Build history of the part. All positions in model axes, mm. Face numbers are marked on the shaded views. A direction names the side the tool comes from. Round coordinates to 2 decimals unless told otherwise and drop trailing zeros. Order: outer loops, then holes, each group sorted by start corner. A loop starts at its lowest first (then second) coordinate and runs counter-clockwise, first axis right, second up. Notation, with made-up numbers: (-19, -22) -> (27, -22) arc R32 ccw to (27, 12) -> close; hole circle Ø7 at (-4, 86). An arc over 180 degrees is marked (long way). Write item = value, one per line.
from build123d import *

# Parameters (mm, degrees)
SKETCH1_W           = 40
SKETCH1_H           = 40
BOSS_EXTRUDE1_DEPTH = 5
CUT_EXTRUDE2_DEPTH  = 39
SKETCH4_W           = 12
SKETCH4_H           = 6.7
CUT_EXTRUDE3_DEPTH  = 29.609264234
SKETCH5_W           = 6
SKETCH5_H           = 6
BOSS_EXTRUDE2_DEPTH = 1.7
FILLET1_R           = 1
SKETCH6_R           = 1
BOSS_EXTRUDE3_DEPTH = 0.5
FILLET2_R           = 1
SKETCH7_R           = 1.6
BOSS_EXTRUDE4_DEPTH = 5
FILLET3_R           = 3


with BuildPart() as part:
    # Sketch1 → Boss-Extrude1 (new body)
    with BuildSketch(Plane(origin=(0, 0, 0), x_dir=(1, 0, 0), z_dir=(0, 1, 0))):
        Rectangle(SKETCH1_W, SKETCH1_H)
    extrude(amount=BOSS_EXTRUDE1_DEPTH)

    # Sketch3 → Cut-Extrude2 (cut)
    with BuildSketch(Plane.XY.offset(20)):
        Polygon((-18.1, 5), (-18.1, 4.2), (-19.1, 4.2), (-19.1, 2.4), (-18.1, 2.4), (-18.1, 0.7), (18.1, 0.7), (18.1, 2.4), (19.1, 2.4), (19.1, 4.2), (18.1, 4.2), (18.1, 5), align=None)
    extrude(amount=-CUT_EXTRUDE2_DEPTH, mode=Mode.SUBTRACT)

    # Sketch4 → Cut-Extrude3 (cut, through all)
    with BuildSketch(Plane(origin=(0, 0.7, 0), x_dir=(1, 0, 0), z_dir=(0, 1, 0))):
        with Locations((8.6, -16.65)):
            Rectangle(SKETCH4_W, SKETCH4_H)
    extrude(amount=-CUT_EXTRUDE3_DEPTH, mode=Mode.SUBTRACT)

    # Sketch5 → Boss-Extrude2 (add)
    with BuildSketch(Plane(origin=(0, 0.7, 0), x_dir=(1, 0, 0), z_dir=(0, 1, 0))):
        with Locations((-15.1, 16)):
            Rectangle(SKETCH5_W, SKETCH5_H)
        with Locations((15.1, 16)):
            Rectangle(SKETCH5_W, SKETCH5_H)
    extrude(amount=BOSS_EXTRUDE2_DEPTH)

    # Fillet1
    fillet1_edges = [part.edges().sort_by_distance(p)[0] for p in [
        (2.6, 0.35, 20),
        (2.6, 0.35, 13.3),
        (14.6, 0.35, 13.3),
        (14.6, 0.35, 20),
        (-18.1, 1.55, -13),
        (-12.1, 1.55, -13),
        (-12.1, 1.55, -19),
        (18.1, 1.55, -13),
        (12.1, 1.55, -19),
        (12.1, 1.55, -13),
    ]]
    fillet(fillet1_edges, radius=FILLET1_R)

    # Sketch6 → Boss-Extrude3 (add)
    with BuildSketch(Plane(origin=(0, 2.4, 0), x_dir=(1, 0, 0), z_dir=(0, 1, 0))):
        with Locations((-17.1, 17)):
            Circle(SKETCH6_R)
        with Locations((17.1, 17)):
            Circle(SKETCH6_R)
    extrude(amount=BOSS_EXTRUDE3_DEPTH)

    # Fillet2
    # the kernel refuses this fillet: 1 mm, written as the material it takes off along each edge
    with BuildSketch(Plane(origin=(-17.1, 2.9, -17), x_dir=(1, 0, 0), z_dir=(0, 0, 1))) as fillet2_piece_1:
        with BuildLine():
            CenterArc((0.133974596, -1), FILLET2_R, 30, 60)
            Line((0.133974596, 0), (0.133974596, 0.02))
            Line((0.133974596, 0.02), (1, 0.02))
            Line((1, 0.02), (1.02, 0))
            ThreePointArc((1.02, 0), (1.02, -0.25), (1.017320508, -0.49))
            Line((1.017320508, -0.49), (1, -0.5))
        make_face()
    revolve(axis=Axis((-17.1, 2.9, -17), (0, 1, 0)), mode=Mode.SUBTRACT)
    with BuildSketch(Plane(origin=(17.1, 2.9, -17), x_dir=(1, 0, 0), z_dir=(0, 0, 1))) as fillet2_piece_2:
        with BuildLine():
            CenterArc((0.133974596, -1), FILLET2_R, 30, 60)
            Line((0.133974596, 0), (0.133974596, 0.02))
            Line((0.133974596, 0.02), (1, 0.02))
            Line((1, 0.02), (1.02, 0))
            ThreePointArc((1.02, 0), (1.02, -0.25), (1.017320508, -0.49))
            Line((1.017320508, -0.49), (1, -0.5))
        make_face()
    revolve(axis=Axis((17.1, 2.9, -17), (0, 1, 0)), mode=Mode.SUBTRACT)

    # Sketch7 → Boss-Extrude4 (add)
    # profile 1 of 2: a face of its own
    with BuildSketch(Plane.XZ):
        with BuildLine():
            Line((-20, 20), (-20, 11.521537766))
            Line((-20, 11.521537766), (-24.997516692, 14.400491632))
            ThreePointArc((-24.997516692, 14.400491632), (-26.398148125, 17.775072543), (-23.5, 20))
            Line((-23.5, 20), (-20, 20))
        make_face()
        with Locations(Location((-23.5, 17, 0), (0, 0, 270))):
            Circle(SKETCH7_R, mode=Mode.SUBTRACT)
    # profile 2 of 2: a face of its own
    with BuildSketch(Plane.XZ):
        with BuildLine():
            Line((20, -20), (20, -11.521537766))
            Line((20, -11.521537766), (24.997516692, -14.400491632))
            ThreePointArc((24.997516692, -14.400491632), (26.398148125, -17.775072543), (23.5, -20))
            Line((23.5, -20), (20, -20))
        make_face()
        with Locations(Location((23.5, -17, 0), (0, 0, 270))):
            Circle(SKETCH7_R, mode=Mode.SUBTRACT)
    extrude(amount=-BOSS_EXTRUDE4_DEPTH)

    # Fillet3
    fillet3_edges = [part.edges().sort_by_distance(p)[0] for p in [
        (-20, 2.5, 11.521537766),
        (20, 2.5, -11.521537766),
    ]]
    fillet(fillet3_edges, radius=FILLET3_R)


solid = part.part
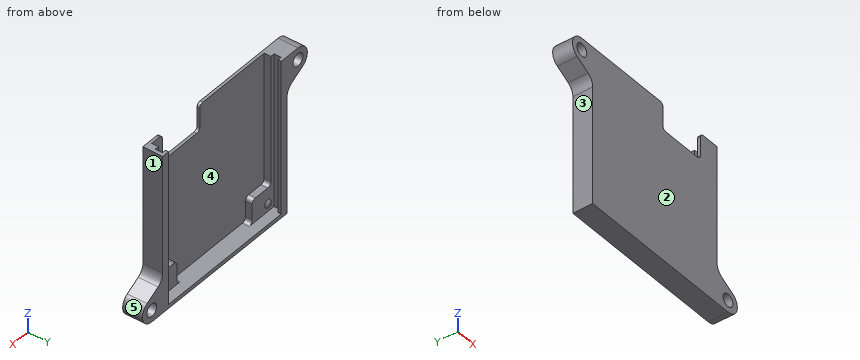
Q1. Which spindle directions (+Z, -Z, +X, -X, +Y, -Y) get a long thin tool onto all of the face, cutting with end or side? Do the marked faces 1, 2, 3, 4 and 5. Say none if no direction does.
Check values:
face_1 = +Z, +X, +Y, -Y
face_2 = +Z, -Z, +X, -X, -Y
face_3 = -Z, -X, +Y, -Y
face_4 = +Z, +Y
face_5 = +X, +Y, -Y
Q2. Cut at D-D, the plane z = -11. List the corners of the cut face in (x, y), and give its area (3 significant figures).
Check values:
outline = (-20, 0) -> (20.26, 0) -> (20.26, 5) -> (18.1, 5) -> (18.1, 4.2) -> (19.1, 4.2) -> (19.1, 2.4) -> (18.1, 2.4) -> (18.1, 0.7) -> (-18.1, 0.7) -> (-18.1, 2.4) -> (-19.1, 2.4) -> (-19.1, 4.2) -> (-18.1, 4.2) -> (-18.1, 5) -> (-20, 5) -> close
area = 42.0 mm²
Q3. Cut at B-B, the plane z = 5.5. List the corners of the cut face in (x, y), and give its area (3 significant figures).
Check values:
outline = (-20, 0) -> (20, 0) -> (20, 5) -> (18.1, 5) -> (18.1, 4.2) -> (19.1, 4.2) -> (19.1, 2.4) -> (18.1, 2.4) -> (18.1, 0.7) -> (-18.1, 0.7) -> (-18.1, 2.4) -> (-19.1, 2.4) -> (-19.1, 4.2) -> (-18.1, 4.2) -> (-18.1, 5) -> (-20, 5) -> close
area = 40.7 mm²
Q4. Cut at A-A, the plane z = 17. List the corners of the cut face in (x, y).
Check values:
outline = (-26.5, 0) -> (-25.1, 0) -> (-25.1, 5) -> (-26.5, 5) -> close; (-21.9, 0) -> (2.6, 0) -> (2.6, 0.7) -> (-18.1, 0.7) -> (-18.1, 2.4) -> (-19.1, 2.4) -> (-19.1, 4.2) -> (-18.1, 4.2) -> (-18.1, 5) -> (-21.9, 5) -> close; (14.6, 0) -> (20, 0) -> (20, 5) -> (18.1, 5) -> (18.1, 4.2) -> (19.1, 4.2) -> (19.1, 2.4) -> (18.1, 2.4) -> (18.1, 0.7) -> (14.6, 0.7) -> close
Q5. Probe probe 1 along X at (y, z) = (4.05, 17); probe 2 along X at (y, z) = (1.65, -17); probe 3 along X at (y, z) = (2, -2). List the from-to ranges inside material, lowest first.
Check values:
probe_1 = -26.5 to -25.1, -21.9 to -19.1, 19.1 to 20
probe_2 = -20 to -12.1, 12.1 to 21.9, 25.1 to 26.5
probe_3 = -20 to -18.1, 18.1 to 20
Q6. Flat gauge pins, fed straight in: pin 1 (1.5 mm diameter, centred on y = 1.5, z = -12, fed in from -X); pin 2 (1.5 mm diameter, centred on y = 2.5, z = 8, fed in from +X); pin 3 (4 mm diameter, centred on x = -11.5, z = 5.5, fed in from +Y). Where does each tip first touch, or does it go through?
Check values:
pin_1 = -20
pin_2 = 20
pin_3 = 0.7
Q7. Cut at C-C, the plane x = 5.5. List the corners of the cut face in (y, z).
Check values:
outline = (0, -20) -> (5, -20) -> (5, -19) -> (0.7, -19) -> (0.7, 13.3) -> (0, 13.3) -> close
